Print and shaded views of the part. All mm, measured from the part's lowest x, y and z. A direction names the side the tool comes from. Round coordinates to 2 decimals unless told otherwise and drop trailing zeros. Loops run counter-clockwise (first coordinate to the right, second up) from the corner with the lowest first, then second, coordinate; pieces in that order, holes last. Notation, with made-up numbers: (37.25, 48) - (64.25, 48) arc R17 cw to (64.25, 71) - close; hole circle Ø10 at (30.5, -11). An arc over 180 degrees is marked (long way). Use one line per item in the form item = value.
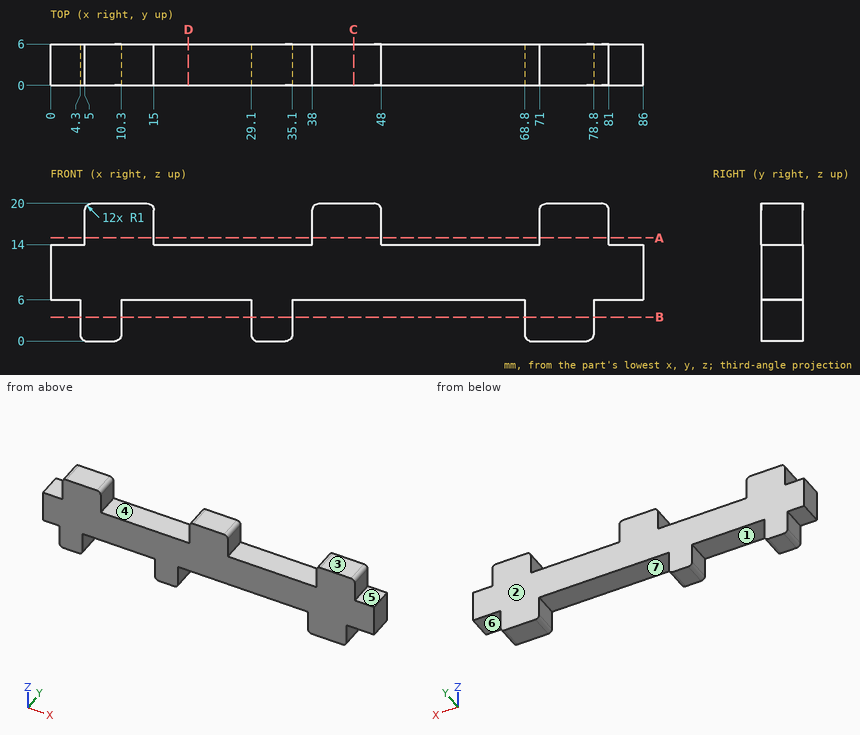
1) Slice it at C-C (x = 44). Write the cut outline in (y, z).
Report:
outline = (0, 6) - (6, 6) - (6, 20) - (0, 20) - close
2) Two-plate mould, pull along X, no slides. Class the marked faces 1 and 2: +X half, -X half, draft (parallel to the pull), parting line (faces both ways), or undercut.
Report:
face_1 = undercut
face_2 = draft
3) Slice it at A-A (z = 15). Write the cut outline in (x, y).
Report:
outline = (5, 0) - (15, 0) - (15, 6) - (5, 6) - close; (38, 0) - (48, 0) - (48, 6) - (38, 6) - close; (71, 0) - (81, 0) - (81, 6) - (71, 6) - close
4) Slice it at D-D (x = 20). Write the cut outline in (y, z), plus the area to 3 significant figures.
Report:
outline = (0, 6) - (6, 6) - (6, 14) - (0, 14) - close
area = 48.0 mm^2
5) Drill centre lines: probe 1 along X at (y, z) = (0.95, 3.75); probe 2 along X at (y, z) = (2, 16); probe 3 along Z at (x, y) = (32, 1.95). Where is each one in solid material? Low to high.
Report:
probe_1 = 4.3 to 10.3, 29.1 to 35.1, 68.8 to 78.8
probe_2 = 5 to 15, 38 to 48, 71 to 81
probe_3 = 0 to 14
6) Tool access for the marked faces 3, 4, 5, 6 and 7: list every direction of +Z, -Z, +X, -X, +Y, -Y with a clear straight run to the whole face (end or side of a thin tool).
Report:
face_3 = +Z, +X, -X, +Y, -Y
face_4 = +Z, +Y, -Y
face_5 = +Z, +X, +Y, -Y
face_6 = -Z, +X, +Y, -Y
face_7 = -Z, +Y, -Y
7) Flat gauge pins, fed straight in: pin 1 (2.5 mm diameter, centred on y = 3, z = 2.5, fed in from -X); pin 2 (3 mm diameter, centred on x = 27, y = 3, fed in from +Z); pin 3 (8 mm diameter, centred on x = 25.5, z = 5.5, fed in from -Y); pin 4 (1.5 mm diameter, centred on y = 3, z = 16, fed in from -X). Where does each tip first touch, or does it go through?
Report:
pin_1 = 4.3
pin_2 = 14
pin_3 = 0
pin_4 = 5
8) Slice it at B-B (z = 3.5). Write the cut outline in (x, y), plus the area to 3 significant figures.
Report:
outline = (4.3, 0) - (10.3, 0) - (10.3, 6) - (4.3, 6) - close; (29.1, 0) - (35.1, 0) - (35.1, 6) - (29.1, 6) - close; (68.8, 0) - (78.8, 0) - (78.8, 6) - (68.8, 6) - close
area = 132 mm^2
